Work out the finished part from the listing and answer in its coordinate system (mm). Face numbers are marked on the shaded views. A direction names the side the tool comes from. Give positions to 0.01 mm unless a question says otherwise; leave off trailing zeros. Write each loop counter-clockwise with the first axis right and the second up, starting at its lowest first coordinate (ties: lowest second). Pieces come first, ordered by that corner, then holes. Notation, with made-up numbers: (-25.75, -34) - (-3.75, -34) arc R23 cw to (-3.75, -14) - close; hole circle Ø3 at (-33.75, 0). An arc over 180 degrees is marked (long way). Write item = value, one per line.
from build123d import *

# Parameters (mm, degrees)
F0_W     = 73.025
F0_H     = 90.588317
F1_DEPTH = 60.325
F0_H_2   = 39.586683
F2_DEPTH = 34.925
F3_W     = 65.405
F3_H     = 53.959612
F4_DEPTH = 3.175
F5_R     = 6.985
F5_R_2   = 4.445
F6_DEPTH = 15.24


with BuildPart() as f1:
    # F0 (on Top) → F1 (new body)
    with BuildSketch(Plane.XY):
        with Locations((0, -19.793341)):
            Rectangle(F0_W, F0_H)
    extrude(amount=F1_DEPTH)

    # F0 (on Top) → F2 (join)
    with BuildSketch(Plane.XY):
        with Locations((0, 45.294158)):
            Rectangle(F0_W, F0_H_2)
        with Locations((0, -19.793341)):
            Rectangle(F0_W, F0_H)
    extrude(amount=F2_DEPTH)

    # F3 (on face) → F4 (join)
    with BuildSketch(Plane.XY.offset(60.325)):
        with Locations((0, -34.297694)):
            Rectangle(F3_W, F3_H)
    extrude(amount=F4_DEPTH)

    # F5 (on face) → F6 (join)
    with BuildSketch(Plane.XY.offset(34.925)):
        with Locations((-18.25625, 51.1175)):
            Circle(F5_R)
        with Locations((0, 39.6875)):
            Circle(F5_R_2)
        with Locations((18.25625, 51.1175)):
            Circle(F5_R)
    extrude(amount=F6_DEPTH)


solid = f1.part
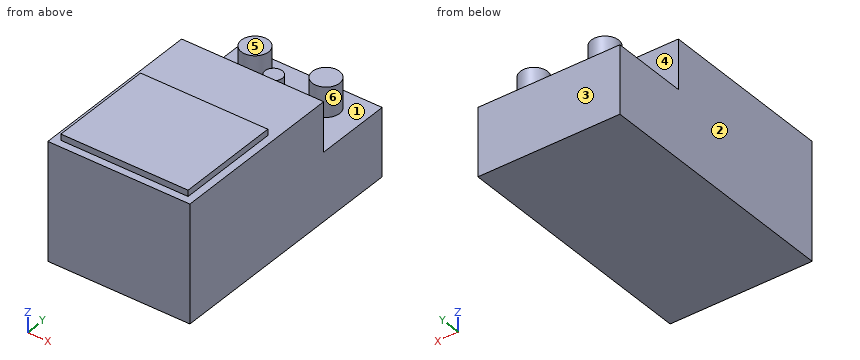
1. Find section B-B, the plane z = 39. Give the vertices of the cut face in (x, y) (1 decimal).
Solution:
outline = (-36.5, -65.1) - (36.5, -65.1) - (36.5, 25.5) - (-36.5, 25.5) - close; circle Ø14 at (-18.3, 51.1); circle Ø8.9 at (0, 39.7); circle Ø14 at (18.3, 51.1)
2. A tool of negligible diameter and unlimited length cuts with its end or side. For the marked faces 4, 5 and 6, from which of +Z, -Z, +X, -X, +Y, -Y can it reach the whole face along a straight path? Write none if from no direction.
Solution:
face_4 = +Z, +X, -X
face_5 = +Z, +X, -X, +Y
face_6 = +Z
3. Find section C-C, the plane y = 8.5. Give the vertices of the cut face in (x, z) (1 decimal), then the cut area to 3 significant figures.
Solution:
outline = (-36.5, 0) - (36.5, 0) - (36.5, 60.3) - (-36.5, 60.3) - close
area = 4,410 mm^2
4. For a pull along Y with two mould halves and no side action, classify the marked faces 1, 2 and 3 as pulls with the +Y half, pulls with the -Y half, needs draft (parallel to the pull), parting line crosses it, or undercut.
Solution:
face_1 = undercut
face_2 = needs draft
face_3 = pulls with the +Y half
5. Find section A-A, the plane x = 8.5. Give the vertices of the cut face in (y, z) (1 decimal).
Solution:
outline = (-65.1, 0) - (65.1, 0) - (65.1, 34.9) - (25.5, 34.9) - (25.5, 60.3) - (-7.3, 60.3) - (-7.3, 63.5) - (-61.3, 63.5) - (-61.3, 60.3) - (-65.1, 60.3) - close
6. Straight lines are drawn through the part: line 1 (Y direction, x = 26.5, z = 37); line 2 (Z direction, x = 33, y = 19) (3 decimals); line 3 (Z direction, x = -7, y = 40) (3 decimals). For each, find the intervals that lie inside material, in ascending order.
Solution:
line_1 = -65.09 to 25.5
line_2 = 0 to 60.325
line_3 = 0 to 34.925
7. Find section D-D, the plane x = 0. Give the vertices of the cut face in (y, z) (1 decimal).
Solution:
outline = (-65.1, 0) - (65.1, 0) - (65.1, 34.9) - (44.1, 34.9) - (44.1, 50.2) - (35.2, 50.2) - (35.2, 34.9) - (25.5, 34.9) - (25.5, 60.3) - (-7.3, 60.3) - (-7.3, 63.5) - (-61.3, 63.5) - (-61.3, 60.3) - (-65.1, 60.3) - close
8. Given pin 1 (1 mm diameter, centred on x = 1.5, z = 62.5, fed in from +Y); pin 2 (4.5 mm diameter, centred on x = 1.5, y = 39.5, fed in from +Z) (3 decimals); pin 3 (1 mm diameter, centred on y = -24.5, z = 62.5, fed in from -X), each flat-ended and moving along its own axis, determine where each tip first touches the part or whether it passes through.
Solution:
pin_1 = -7.32
pin_2 = 50.165
pin_3 = -32.7
